The model under review builds one solid part; all positions refer to its coordinate system, in mm. Face numbers are marked on the shaded views. A direction names the side the tool comes from. Give positions to 0.01 mm unless a question says otherwise; leave off trailing zeros. Order: outer loops, then holes, each group sorted by start corner. A loop starts at its lowest first (then second) coordinate and runs counter-clockwise, first axis right, second up. Notation, with made-up numbers: (73.25, 7.25) - (102.25, 7.25) arc R8 ccw to (102.25, 16.25) - close; hole circle Ø11 at (38, -17.75). An arc over 180 degrees is marked (long way). Use CSV: the item, a comma, the result in double quotes. Start each with the question number.
1. Take a section at D-D, the plane z = -11. State the section outline as (x, y) points, then the cut area to 3 significant figures.
2. Draft analysis for pull direction Y (two halves, no side actions). For the marked faces 1, 2, 3 and 4, state which applies: released by +Y, released by -Y, zero draft, split by the parting line, or undercut.
3. For pin 1 (5 mm diameter, centred on x = 13, z = -47, fed in from -Y); pin 2 (9.5 mm diameter, centred on y = -87.5, z = 15.5, fed in from -X); pin 3 (10 mm diameter, centred on x = 0, z = 42, fed in from +Y), all flat-tipped, find the tip position at first contact; note any pin that passes through.
4. Take a section at B-B, the plane y = 57.5. State the section outline as (x, z) points, then the cut area to 3 significant figures.
5. To check wall thickness, follow line 1 (X direction, y = 109, z = 42); line 2 (Z direction, x = 5, y = -70); line 3 (Z direction, x = 13, y = 22). State the ranges of each line that lie inside material, in increasing order. Write a range as [from, to].
6. Take a section at A-A, the plane x = 0. Count the separate pieces of the cut face and the enclosed holes in it, then the cut area to 3 significant figures.
7. Take a section at C-C, the plane x = -17. State the section outline as (y, z) points.
8. Machinability: for the marked faces 5, 6 and 7, which of the approach directions +Z, -Z, +X, -X, +Y, -Y give a long, thin tool a straight path to every point of the face, cutting with its end or side? Answer none if there is none.
```python
from build123d import *

# Parameters (mm, degrees)
BOSS_EXTRUDE1_DEPTH = 20
BOSS_EXTRUDE2_DEPTH = 20
CUT_EXTRUDE1_DEPTH  = 40
SKETCH3_R           = 6.35
CUT_EXTRUDE2_DEPTH  = 40
BOSS_EXTRUDE3_DEPTH = 20
SKETCH6_R           = 6.35
CUT_EXTRUDE4_DEPTH  = 40
SKETCH9_R           = 30
SKETCH9_R_2         = 23.625
BOSS_EXTRUDE4_DEPTH = 15
SKETCH9_3_R         = 23.625
SKETCH9_3_R_2       = 22.5
BOSS_EXTRUDE5_DEPTH = 25
SKETCH9_4_R         = 22.5
SKETCH9_4_R_2       = 20.075
BOSS_EXTRUDE6_DEPTH = 70
SKETCH9_5_R         = 20.075
SKETCH9_5_R_2       = 14.175
BOSS_EXTRUDE7_DEPTH = 80
SKETCH9_6_R         = 14.175
BOSS_EXTRUDE8_DEPTH = 120
CUT_EXTRUDE5_DEPTH  = 120
SKETCH12_R          = 6.35
BOSS_EXTRUDE9_DEPTH = 7.5


with BuildPart() as part:
    # Sketch1 → Boss-Extrude1 (new body)
    with BuildSketch(Plane.XY):
        with BuildLine():
            Line((20, 80), (-20, 80))
            Line((-20, 80), (-20, 40.311288741))
            ThreePointArc((-20, 40.311288741), (0, 45), (20, 40.311288741))
            Line((20, 40.311288741), (20, 80))
        make_face()
        with BuildLine():
            ThreePointArc((20, 40.311288741), (0, 45), (-20, 40.311288741))
            Line((-20, 40.311288741), (-20, -40.311288741))
            ThreePointArc((-20, -40.311288741), (0, -45), (20, -40.311288741))
            Line((20, -40.311288741), (20, 40.311288741))
        make_face()
        with BuildLine():
            ThreePointArc((45, 0), (38.242646352, 23.717082451), (20, 40.311288741))
            Line((20, 40.311288741), (20, -40.311288741))
            ThreePointArc((20, -40.311288741), (38.242646352, -23.717082451), (45, 0))
        make_face()
        with BuildLine():
            ThreePointArc((20, -40.311288741), (0, -45), (-20, -40.311288741))
            Line((-20, -40.311288741), (-20, -80))
            Line((-20, -80), (20, -80))
            Line((20, -80), (20, -40.311288741))
        make_face()
        with BuildLine():
            Line((-20, -40.311288741), (-20, 40.311288741))
            ThreePointArc((-20, 40.311288741), (-45, 0), (-20, -40.311288741))
        make_face()
    extrude(amount=BOSS_EXTRUDE1_DEPTH)

    # Sketch2 → Boss-Extrude2 (add, symmetric)
    with BuildSketch(Plane(origin=(0, 0, 0), x_dir=(0, 0, -1), z_dir=(1, 0, 0))):
        Polygon((-20, 80), (0, 80), (-9.116936514, 117.5), (-63.916468616, 117.5), (-63.916468616, 102.5), (-25.470161908, 102.5), align=None)
    extrude(amount=BOSS_EXTRUDE2_DEPTH, both=True)

    # Sketch4 → Cut-Extrude1 (cut)
    with BuildSketch(Plane(origin=(0, 117.5, 0), x_dir=(1, 0, 0), z_dir=(0, 1, 0))):
        with BuildLine():
            Line((-20, -42), (-20, -63.916468616))
            Line((-20, -63.916468616), (20, -63.916468616))
            Line((20, -63.916468616), (20, -42))
            ThreePointArc((20, -42), (0, -62), (-20, -42))
        make_face()
    extrude(amount=-CUT_EXTRUDE1_DEPTH, mode=Mode.SUBTRACT)

    # Sketch3 → Cut-Extrude2 (cut)
    with BuildSketch(Plane(origin=(0, 117.5, 0), x_dir=(1, 0, 0), z_dir=(0, 1, 0))):
        with Locations((0, -42)):
            Circle(SKETCH3_R)
    extrude(amount=-CUT_EXTRUDE2_DEPTH, mode=Mode.SUBTRACT)

    # Sketch5 → Boss-Extrude3 (add, symmetric)
    with BuildSketch(Plane(origin=(0, 0, 0), x_dir=(0, 0, -1), z_dir=(1, 0, 0))):
        Polygon((-20, -80), (0, -80), (-4.065810475, -116.5), (-57.146175878, -116.5), (-57.146175878, -101.5), (-22.394929458, -101.5), align=None)
    extrude(amount=BOSS_EXTRUDE3_DEPTH, both=True)

    # Sketch6 → Cut-Extrude4 (cut)
    with BuildSketch(Plane.XZ.offset(116.5)):
        with Locations((0, 31.3)):
            Circle(SKETCH6_R)
    extrude(amount=-CUT_EXTRUDE4_DEPTH, mode=Mode.SUBTRACT)

    # Sketch9 → Boss-Extrude4 (add)
    with BuildSketch(Plane(origin=(0, 0, 0), x_dir=(-1, 0, 0), z_dir=(0, 0, -1))):
        Circle(SKETCH9_R)
        Circle(SKETCH9_R_2, mode=Mode.SUBTRACT)
    extrude(amount=BOSS_EXTRUDE4_DEPTH)

    # Sketch9_3 → Boss-Extrude5 (add)
    with BuildSketch(Plane(origin=(0, 0, 0), x_dir=(-1, 0, 0), z_dir=(0, 0, -1))):
        Circle(SKETCH9_3_R)
        Circle(SKETCH9_3_R_2, mode=Mode.SUBTRACT)
    extrude(amount=BOSS_EXTRUDE5_DEPTH)

    # Sketch9_4 → Boss-Extrude6 (add)
    with BuildSketch(Plane(origin=(0, 0, 0), x_dir=(-1, 0, 0), z_dir=(0, 0, -1))):
        Circle(SKETCH9_4_R)
        Circle(SKETCH9_4_R_2, mode=Mode.SUBTRACT)
    extrude(amount=BOSS_EXTRUDE6_DEPTH)

    # Sketch9_5 → Boss-Extrude7 (add)
    with BuildSketch(Plane(origin=(0, 0, 0), x_dir=(-1, 0, 0), z_dir=(0, 0, -1))):
        Circle(SKETCH9_5_R)
        Circle(SKETCH9_5_R_2, mode=Mode.SUBTRACT)
    extrude(amount=BOSS_EXTRUDE7_DEPTH)

    # Sketch9_6 → Boss-Extrude8 (add)
    with BuildSketch(Plane(origin=(0, 0, 0), x_dir=(-1, 0, 0), z_dir=(0, 0, -1))):
        Circle(SKETCH9_6_R)
    extrude(amount=BOSS_EXTRUDE8_DEPTH)

    # Sketch10 → Cut-Extrude5 (cut)
    with BuildSketch(Plane(origin=(0, -101.5, 0), x_dir=(1, 0, 0), z_dir=(0, 1, 0))):
        with BuildLine():
            Line((-20, -31.3), (-20, -57.146175878))
            Line((-20, -57.146175878), (20, -57.146175878))
            Line((20, -57.146175878), (20, -31.3))
            ThreePointArc((20, -31.3), (0, -51.3), (-20, -31.3))
        make_face()
    extrude(amount=-CUT_EXTRUDE5_DEPTH, mode=Mode.SUBTRACT)

    # Sketch12 → Boss-Extrude9 (add, symmetric)
    with BuildSketch(Plane(origin=(0, 0, 0), x_dir=(1, 0, 0), z_dir=(0, 1, 0))):
        with BuildLine():
            Line((45, -2.018705138), (44.876123934, -17.463703547))
            add(Edge.make_bspline(
                [(44.876123934, -17.463703547), (53.437219623, -24.801983569), (60.835955623, -31.879035395)],
                knots=[0, 0, 0, 1, 1, 1], degree=2))
            ThreePointArc((60.835955623, -31.879035395), (72.992020693, -26.306274296), (68.799253388, -13.607995414))
            add(Edge.make_bspline(
                [(45, -2.018705138), (59.856089875, -6.764812241), (68.799253388, -13.607995414)],
                knots=[0, 0, 0, 1, 1, 1], degree=2))
        make_face()
        with Locations((63.8, -22.3)):
            Circle(SKETCH12_R, mode=Mode.SUBTRACT)
    extrude(amount=BOSS_EXTRUDE9_DEPTH, both=True)


solid = part.part
```
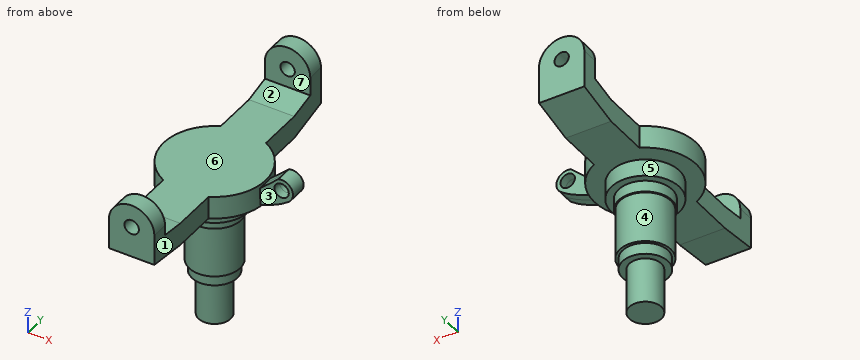
Determined:
1,outline,"circle Ø60 at (0, 0)"
1,area,"2,830 mm²"
2,face 1,"zero draft"
2,face 2,"undercut"
2,face 3,"released by -Y"
2,face 4,"split by the parting line"
3,pin 1,"stops at y = -19.9"
3,pin 2,"stops at x = -20"
3,pin 3,"stops at y = -101.5"
4,outline,"(-20, 0) - (20, 0) - (20, 20) - (-20, 20) - close"
4,area,"800 mm²"
5,line 1,"x = [-20, -6.35], [6.35, 20]"
5,line 2,"z = [0, 20]"
5,line 3,"z = [-15, 20]"
6,separate pieces,"3"
6,enclosed holes,"0"
6,area,"10,200 mm²"
7,outline,"(-116.5, 4.07) - (-80, 0) - (-24.72, 0) - (-24.72, -15) - (-16.41, -15) - (-16.41, -25) - (-14.74, -25) - (-14.74, -70) - (-10.68, -70) - (-10.68, -80) - (10.68, -80) - (10.68, -70) - (14.74, -70) - (14.74, -25) - (16.41, -25) - (16.41, -15) - (24.72, -15) - (24.72, 0) - (80, 0) - (117.5, 9.12) - (117.5, 52.54) - (102.5, 52.54) - (102.5, 25.47) - (80, 20) - (-80, 20) - (-101.5, 22.39) - (-101.5, 41.84) - (-116.5, 41.84) - close"
8,face 5,"-Z"
8,face 6,"+Z, -X"
8,face 7,"+Z, +X, -X"
